Autodesk Inventor part; units mm, degrees
ref_plane "作業平面1" through (0, 29.35, 0) normal (0, 1, 0) x (1, 0, 0)
ref_plane "YZ Plane" through (0, 0, 0) normal (1, 0, 0) x (0, 1, 0)
ref_plane "XZ Plane" through (0, 0, 0) normal (0, 1, 0) x (-1, 0, 0)
sketch "スケッチ1" plane through (0, 0, 0) normal (0, 1, 0) x (-1, 0, 0)
  line L0 (0, 0) -> (12, 0)
  line L1 (12, 0) -> (12, -23.3)
  line L2 (12, -23.3) -> (0, -23.3)
  line L3 (0, -23.3) -> (0, 0)
  dimension "d0" = 23.3
  dimension "d1" = 12
extrude "押し出し1" add sketch "スケッチ1" along normal blind 18.45
sketch "スケッチ2" plane through (0, 18.45, 0) normal (0, 1, 0) x (1, 0, 0)
  circle A0 centre (-6, 17.3) radius 6
  line L0 (-12, 23.3) -> (-12, 0)
  line L1 (0, 0) -> (0, 23.3)
  line L2 (0, 23.3) -> (-12, 23.3)
  circle A1 centre (-6, 11.6) radius 2.5
  line L3 (-7.973197, 10.064912) -> (-10.735672, 13.615789)
  line L4 (-4.026803, 10.064912) -> (-1.264328, 13.615789)
  point P0 (-8.488419, 11.840351)
  point P1 (-3.511581, 11.840351)
  dimension "d20" = 5.7
  dimension "d21" = 5
extrude "押し出し2" add sketch "スケッチ2" along normal blind 6.9 contours A0 A1 | L4 A1 A0 | A1 A0 | A0 A1 | A1 L3 A0
sketch "スケッチ3" plane through (-6, 25.35, -17.3) normal (0, 1, 0) x (-1, 0, 0)
  arc A0 (-4.735672, 3.684211) -> (4.735672, 3.684211) centre (0, 0) ccw
  circle A1 centre (0, 0) radius 2.5
  point P0 (-6, 17.3)
  point P1 (-2.386497, 4.955263)
  point P2 (2.386497, 4.955263)
  dimension "d6" = 5
extrude "押し出し3" add sketch "スケッチ3" along normal blind 3.1
sketch "スケッチ4" plane through (0, 18.45, 0) normal (0, 1, 0) x (1, 0, 0)
  line L0 (0, 0) -> (0, 23.3)
  line L1 (0, 17.3) -> (0, 23.3)
  line L2 (0, 0) -> (0, 17.3)
  line L3 (0, 23.3) -> (-12, 23.3)
  line L4 (0, 0) -> (0, 23.3)
  line L5 (-12, 0) -> (0, 0)
  line L6 (-12, 23.3) -> (-12, 0)
  line L7 (-12, -4.6) -> (0, -4.6)
  line L8 (0, -4.6) -> (0, 27.9)
  line L9 (0, 27.9) -> (-12, 27.9)
  line L10 (-12, 27.9) -> (-12, -4.6)
  line L11 (-12, -2.6) -> (0, -2.6) construction
  line L12 (0, -2.6) -> (0, 25.9) construction
  line L13 (0, 25.9) -> (-12, 25.9) construction
  line L14 (-12, 25.9) -> (-12, -2.6) construction
  line L15 (0, 17.3) -> (0, 23.3)
  circle A0 centre (-6, -2.6) radius 0.85
  circle A1 centre (-6, 25.9) radius 0.85
  point P0 (-12, 11.65)
  point P1 (-12, 23.3)
  dimension "d9" = 32.5
  dimension "d10" = 28.5
  dimension "d11" = 1.7
  dimension "d12" = 1.7
extrude "押し出し4" add sketch "スケッチ4" against normal blind 1.6 contours L8 L7 L10 L5 | L3 L10 L9 L8
sketch "スケッチ5" plane through (0, 18.45, 0) normal (0, 1, 0) x (1, 0, 0)
  line L0 (0, 23.3) -> (-12, 23.3)
  line L1 (0, 0) -> (0, 23.3)
  line L2 (-12, 0) -> (0, 0)
  line L3 (-12, 23.3) -> (-12, 0)
extrude "押し出し5" add sketch "スケッチ5" along normal blind 3.1
chamfer "面取り1" distance 8 distance2 2 1 edges at (-6, 21.55, 0) measured on face at (-6, 21.55, -3.0333)
ref_plane "作業平面1" through (0, 29.35, 0) normal (0, 1, 0) x (1, 0, 0)
sketch "スケッチ6" plane through (0, 29.35, 0) normal (0, 1, 0) x (1, 0, 0)
  circle A0 centre (-6, 17.3) radius 2.5
  circle A1 centre (-6, 17.3) radius 11.9
  circle A2 centre (-6, 27.2) radius 2
  circle A3 centre (-15.9, 17.3) radius 2
  circle A4 centre (-6, 7.4) radius 2
  circle A5 centre (3.9, 17.3) radius 2
  line L0 (4.00101, 19.297448) -> (-5.873737, 19.79681)
  line L1 (-5.873737, 14.80319) -> (4.00101, 15.302552)
  line L2 (-7.997448, 27.30101) -> (-8.49681, 17.426263)
  line L3 (-3.50319, 17.426263) -> (-4.002552, 27.30101)
  line L4 (-16.00101, 15.302552) -> (-6.126263, 14.80319)
  line L5 (-6.126263, 19.79681) -> (-16.00101, 19.297448)
  line L6 (-4.002552, 7.29899) -> (-3.50319, 17.173737)
  line L7 (-8.49681, 17.173737) -> (-7.997448, 7.29899)
  point P0 (0, 0)
  point P1 (-8.382702, 14.917298)
  point P2 (-7.997448, 7.29899)
  point P3 (-4.002552, 7.29899)
  point P4 (-3.617298, 14.917298)
  point P5 (-3.617298, 19.682702)
  point P6 (-4.002552, 27.30101)
  point P7 (-7.997448, 27.30101)
  point P8 (-8.382702, 19.682702)
  point P9 (-16.00101, 19.297448)
  dimension "d34" = 23.8
  dimension "d35" = 4
  dimension "d38" = 360
  dimension "d42" = 360
sketch "スケッチ6 outline for 押し出し6" plane through (0, 29.35, 0) normal (0, 1, 0) x (1, 0, 0)
  line L0 (-8.382702, 14.917298) -> (-7.997448, 7.29899)
  arc A0 (-7.997448, 7.29899) -> (-4.002552, 7.29899) centre (-6, 7.4) ccw
  line L1 (-4.002552, 7.29899) -> (-3.617298, 14.917298)
  line L2 (-3.617298, 14.917298) -> (4.00101, 15.302552)
  arc A1 (4.00101, 15.302552) -> (4.00101, 19.297448) centre (3.9, 17.3) ccw
  line L3 (4.00101, 19.297448) -> (-3.617298, 19.682702)
  line L4 (-3.617298, 19.682702) -> (-4.002552, 27.30101)
  arc A2 (-4.002552, 27.30101) -> (-7.997448, 27.30101) centre (-6, 27.2) ccw
  line L5 (-7.997448, 27.30101) -> (-8.382702, 19.682702)
  line L6 (-8.382702, 19.682702) -> (-16.00101, 19.297448)
  arc A3 (-16.00101, 19.297448) -> (-16.00101, 15.302552) centre (-15.9, 17.3) ccw
  line L7 (-16.00101, 15.302552) -> (-8.382702, 14.917298)
extrude "押し出し6" add sketch "スケッチ6 outline for 押し出し6" against normal blind 1.6
sketch "スケッチ7" plane through (0, 29.35, 0) normal (0, 1, 0) x (1, 0, 0)
  circle A0 centre (-6, 17.3) radius 2.5
  circle A1 centre (-6, 17.3) radius 2.95
  point P0 (0, 0)
  dimension "d46" = 5.9
extrude "押し出し7" add sketch "スケッチ7" along normal blind 0.8 contours A0 | A1
properties part number "FT90MR" material "ABS プラスチック"
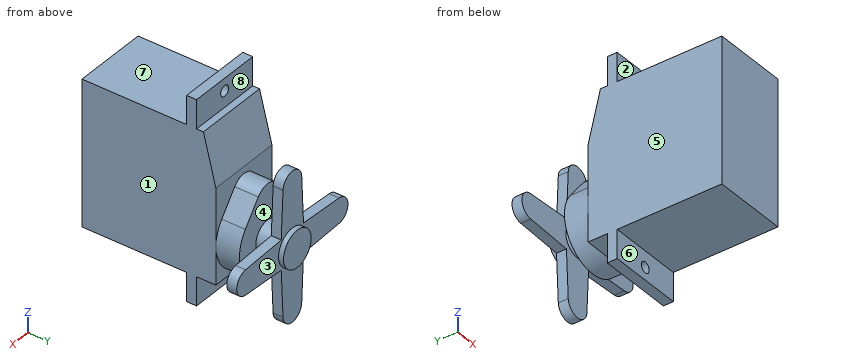
CAD build for the part. Positions are in the model's coordinates, mm. Face numbers are marked on the shaded views. A direction names the side the tool comes from. Round coordinates to 2 decimals unless told otherwise and drop trailing zeros. Order: outer loops, then holes, each group sorted by start corner. A loop starts at its lowest first (then second) coordinate and runs counter-clockwise, first axis right, second up. Notation, with made-up numbers: (74.5, 76.25) - (99.5, 76.25) arc R18 cw to (99.5, 101.25) - close; hole circle Ø10 at (39.25, 75). An arc over 180 degrees is marked (long way). Answer in a Markdown table with one row per item. Add a question column.
(1) 3-axis set-ups, long thin cutter, end or side, ignore diameter. For the marked faces 5, 6, 7 and 8: which of +Z, -Z, +X, -X, +Y, -Y reach the whole face in a straight line?
(2) Band-saw the part on C-C on z = -25.9. List the corners of the cut face in (x, y).
(3) Band-saw the part on D-D on y = 5. List the corners of the cut face in (x, z), and give its area (3 significant figures).
(4) Mould opens along Y. For the marked faces 1, 2, 3 and 4 say: +Y half, -Y half, draft (parallel to the pull), parting line (faces both ways), or undercut.
(5) Band-saw the part on B-B on x = -10.25. List the corners of the cut face in (y, z).
(6) Drop flat-ended pins along their axis: pin 1 Ø2 at (y, z) = (12, -22) entering from -X; pin 2 Ø3 at (x, z) = (-8, -5.5) entering from +Y; pin 3 Ø8 at (x, y) = (-9.5, 26.5) entering from +Z. Give the stop position or say it passes through.
(7) Band-saw the part on A-A on z = 2.6. List the corners of the cut face in (x, y).
(8) Probe L1, parallel to Z at x = -6, y = 17.3; L2, parallel to X at y = 17.5, z = -23.5; L3, parallel to Y at x = -10, z = -19. List the from-to ranges inside material, lowest first. Write a range as [from, to].
Data:
| question | item | result |
|---|---|---|
| 1 | face 5 | +Z, -Z, -X, -Y |
| 1 | face 6 | -Z, +X, -X, -Y |
| 1 | face 7 | +Z, +X, -X, -Y |
| 1 | face 8 | +Z, +X, -X, +Y |
| 2 | outline | (-12, 16.85) - (-6.85, 16.85) - (-6.85, 18.45) - (-12, 18.45) - close; (-8.07, 27.75) - (-3.93, 27.75) - (-3.93, 29.35) - (-8.07, 29.35) - close; (-5.15, 16.85) - (0, 16.85) - (0, 18.45) - (-5.15, 18.45) - close |
| 3 | outline | (-12, -23.3) - (0, -23.3) - (0, 0) - (-12, 0) - close |
| 3 | area | 280 mm^2 |
| 4 | face 1 | draft |
| 4 | face 2 | -Y half |
| 4 | face 3 | +Y half |
| 4 | face 4 | undercut |
| 5 | outline | (0, -23.3) - (16.85, -23.3) - (16.85, -27.9) - (18.45, -27.9) - (18.45, -23.3) - (21.55, -23.3) - (21.55, -21.54) - (25.35, -21.54) - (25.35, -12.99) - (21.55, -12.99) - (21.55, -8) - (19.55, 0) - (18.45, 0) - (18.45, 4.6) - (16.85, 4.6) - (16.85, 0) - (0, 0) - close; (27.75, -19.59) - (29.35, -19.59) - (29.35, -15.01) - (27.75, -15.01) - close |
| 6 | pin 1 | stops at x = -12 |
| 6 | pin 2 | stops at y = 29.35 |
| 6 | pin 3 | stops at z = -5.4 |
| 7 | outline | (-12, 16.85) - (-6.85, 16.85) - (-6.85, 18.45) - (-12, 18.45) - close; (-5.15, 16.85) - (0, 16.85) - (0, 18.45) - (-5.15, 18.45) - close |
| 8 | L1 | z = [-27.9, -26.75], [-25.05, 1.75], [3.45, 4.6] |
| 8 | L2 | x = [-12, 0] |
| 8 | L3 | y = [0, 25.35], [27.75, 29.35] |
